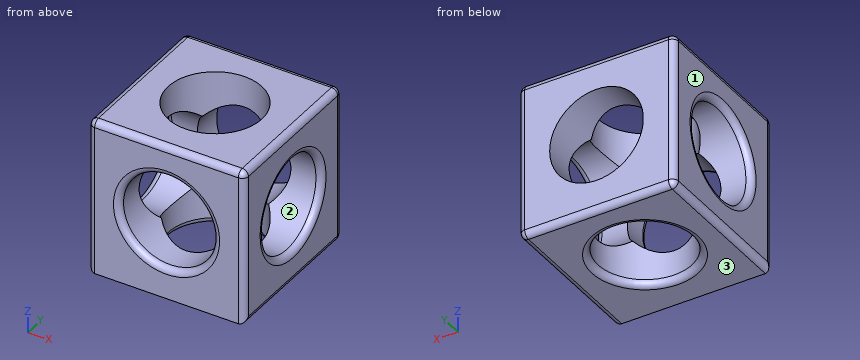
from build123d import *

# Parameters (mm, degrees)
F0_W     = 127
F0_H     = 127
F1_DEPTH = 127
F2_R     = 38.1
F3_DEPTH = 127
F4_R     = 38.1
F5_DEPTH = 127
F6_R     = 38.1
F7_DEPTH = 127
F8_R     = 5.08


with BuildPart() as f1:
    # F0 (on Top) → F1 (new body)
    with BuildSketch(Plane.XY):
        with Locations((5.959775, -5.865746)):
            Rectangle(F0_W, F0_H)
    extrude(amount=F1_DEPTH)

    # F2 (on face) → F3 (cut)
    with BuildSketch(Plane(origin=(-57.540225, 0, 0), x_dir=(0, -1, 0), z_dir=(-1, 0, 0))):
        with Locations((5.865746, 63.5)):
            Circle(F2_R)
    extrude(amount=-F3_DEPTH, mode=Mode.SUBTRACT)

    # F4 (on face) → F5 (cut)
    with BuildSketch(Plane.XZ.offset(69.365746)):
        with Locations((5.959775, 63.5)):
            Circle(F4_R)
    extrude(amount=-F5_DEPTH, mode=Mode.SUBTRACT)

    # F6 (on face) → F7 (cut)
    with BuildSketch(Plane(origin=(0, 0, 0), x_dir=(1, 0, 0), z_dir=(0, 0, -1))):
        with Locations((5.959775, 5.865746)):
            Circle(F6_R)
    extrude(amount=-F7_DEPTH, mode=Mode.SUBTRACT)

    # F8
    f8_edges = [f1.edges().sort_by_distance(p)[0] for p in [
        (-57.540225, 57.634254, 63.5),
        (5.959775, 57.634254, 0),
        (69.459775, 57.634254, 63.5),
        (5.959775, 57.634254, 127),
        (-57.540225, -5.865746, 0),
        (-57.540225, -69.365746, 63.5),
        (-57.540225, -5.865746, 127),
        (5.959775, -69.365746, 127),
        (69.459775, -5.865746, 127),
        (69.459775, -5.865746, 0),
        (69.459775, -69.365746, 63.5),
        (69.459775, 32.234254, 63.5),
        (-32.140225, -5.865746, 0),
        (-57.540225, 32.234254, 63.5),
        (-32.140225, -69.365746, 63.5),
    ]]
    fillet(f8_edges, radius=F8_R)


solid = f1.part
Design review of the part built by this model. Coordinates are the model's own, in mm. Face numbers are marked on the shaded views. Coordinates: 2 decimals unless noted, no trailing zeros. Write each loop counter-clockwise with the first axis right and the second up, starting at its lowest first coordinate (ties: lowest second). Pieces come first, ordered by that corner, then holes. Notation, with made-up numbers: (10, 33.5) - (53, 33.5) arc R30 cw to (53, 60.5) - close; hole circle Ø5 at (6.5, 4.25). An arc over 180 degrees is marked (long way). Use one line per item in the form item = value.
Q1. Insertion check: pin 1 Ø1 at (x, z) = (44, 81.5) entering from -Y; pin 2 Ø1.5 at (x, z) = (-20, 31.5) entering from -Y; pin 3 Ø1.5 at (x, y) = (23.5, 26) entering from +Z; pin 4 Ø3 at (x, y) = (12.5, -44.5) entering from -Z. Each pin has a flat end and moves straight along its axis. Give the tip position at first contact, or say it passes through.
Taken from the geometry:
pin_1 = -69.33
pin_2 = -69.22
pin_3 = through
pin_4 = 0.66
Q2. For probe 1 along X at (y, z) = (-6, 11.5); probe 2 along Z at (x, y) = (45, 6); probe 3 along Y at (x, z) = (-19, 112.5), list the stretches that pass through material, from the lowest coordinate up.
Taken from the geometry:
probe_1 = -57.54 to -32.14, 44.06 to 69.46
probe_2 = 0.59 to 27.29, 99.71 to 127
probe_3 = -69.37 to -34.65, 22.92 to 57.63
Q3. Consider section A-A (z = 63.5). Write out the cut boundary in (x, y).
Taken from the geometry:
outline = (-57.54, -64.29) arc R5.08 ccw to (-52.46, -69.37) - (-37.22, -69.37) arc R5.08 ccw to (-32.14, -64.29) - (-32.14, -43.97) - (-52.46, -43.97) arc R5.08 ccw to (-57.54, -49.05) - close; (-57.54, 37.31) arc R5.08 ccw to (-52.46, 32.23) - (-32.14, 32.23) - (-32.14, 57.63) - (-52.46, 57.63) arc R5.08 ccw to (-57.54, 52.55) - close; (44.06, -64.29) arc R5.08 ccw to (49.14, -69.37) - (64.38, -69.37) arc R5.08 ccw to (69.46, -64.29) - (69.46, -49.05) arc R5.08 ccw to (64.38, -43.97) - (44.06, -43.97) - close; (44.06, 32.23) - (64.38, 32.23) arc R5.08 ccw to (69.46, 37.31) - (69.46, 52.55) arc R5.08 ccw to (64.38, 57.63) - (44.06, 57.63) - close
Q4. The part is to be moulded in two halves that separate along Z. For the marked faces 1, 2 and 3, say which applies: +Z half, -Z half, draft (parallel to the pull), parting line (faces both ways), or undercut.
Taken from the geometry:
face_1 = draft
face_2 = undercut
face_3 = -Z half
Q5. Consider section B-B (x = -3). Count the separate pieces of the cut face and the enclosed holes in it, plus the area to 3 significant figures.
Taken from the geometry:
separate_pieces = 4
enclosed_holes = 0
area = 2,760 mm^2
